Design review of the part built by this model. Coordinates are the model's own, in mm. A direction names the side the tool comes from. Coordinates: 2 decimals unless noted, no trailing zeros. Order: outer loops, then holes, each group sorted by start corner. A loop starts at its lowest first (then second) coordinate and runs counter-clockwise, first axis right, second up. Notation, with made-up numbers: (-6.5, 83) -> (-2.5, 83) arc R20 ccw to (-2.5, 96) -> close; hole circle Ø6 at (27, -20). An arc over 180 degrees is marked (long way). Write item = value, one per line.
```python
from build123d import *

# Parameters (mm, degrees)
F0_W      = 44
F0_H      = 27
F1_DEPTH  = 9
F2_W      = 34
F2_H      = 23
F3_DEPTH  = 7
F6_W      = 6
F6_H      = 7.5
F7_DEPTH  = 4
F5_W      = 6
F5_H      = 7.5
F10_DEPTH = 4
F12_DEPTH = 5
F14_R     = 2
F15_R     = 5


with BuildPart() as f1:
    # F0 (on Top) → F1 (new body)
    with BuildSketch(Plane.XY):
        with Locations((-1, 0)):
            Rectangle(F0_W, F0_H)
    extrude(amount=-F1_DEPTH)


with BuildPart() as f3:
    # F2 (on Top) → F3 (new body)
    with BuildSketch(Plane.XY):
        with Locations((4, 0)):
            Rectangle(F2_W, F2_H)
    extrude(amount=-F3_DEPTH)


with BuildPart() as f1_1:
    add(f1.part)

    # F4: cut F3
    add(f3.part, mode=Mode.SUBTRACT)


with BuildPart() as f7:
    # F6 (on Top) → F7 (new body)
    with BuildSketch(Plane.XY):
        with Locations((-16, -7.75)):
            Rectangle(F6_W, F6_H)
    extrude(amount=-F7_DEPTH)


with BuildPart() as f7b:
    # F5 (on Top) → F7, piece 2 (new body)
    with BuildSketch(Plane.XY):
        with Locations((-16, 7.75)):
            Rectangle(F5_W, F5_H)
    extrude(amount=-F7_DEPTH)


with BuildPart() as f1_2:
    add(f1_1.part)

    # F8: cut F7b, F7
    add(f7b.part, mode=Mode.SUBTRACT)
    add(f7.part, mode=Mode.SUBTRACT)

    # F9 (on face) → F10 (join)
    with BuildSketch(Plane(origin=(-23, 0, 0), x_dir=(0, -1, 0), z_dir=(-1, 0, 0))):
        Polygon((-13.5, 0), (13.5, 0), (33.5, 34.6410161514), (-33.5, 34.6410161514), align=None)
    extrude(amount=-F10_DEPTH)


with BuildPart() as f12:
    # F11 (on face) → F12 (new body)
    with BuildSketch(Plane(origin=(-23, 0, 0), x_dir=(0, -1, 0), z_dir=(-1, 0, 0))):
        Polygon((-7.5, 0), (7.5, 0), (27.5, 34.6410161514), (-27.5, 34.6410161514), align=None)
    extrude(amount=-F12_DEPTH)


with BuildPart() as f1_3:
    add(f1_2.part)

    # F13: cut F12
    add(f12.part, mode=Mode.SUBTRACT)

    # F14
    f14_edges = [f1_3.edges().sort_by_distance(p)[0] for p in [
        (-21, 33.5, 34.641016),
        (-21, 27.5, 34.641016),
        (-21, -27.5, 34.641016),
        (-21, -33.5, 34.641016),
        (-21, -7.5, 0),
        (-21, 7.5, 0),
        (-13, 0, 0),
        (-13, 7.75, -4),
        (-13, -7.75, -4),
    ]]
    fillet(f14_edges, radius=F14_R)

    # F15
    f15_edges = [f1_3.edges().sort_by_distance(p)[0] for p in [
        (-19, -12.5, 0),
        (-19, 12.5, 0),
        (21, 12.5, 0),
        (21, -12.5, 0),
    ]]
    fillet(f15_edges, radius=F15_R)


solid = f1_3.part
```
(1) Insertion check: pin 1 (1.6 mm diameter, centred on x = -4, y = -13, fed in from +Z); pin 2 (3 mm diameter, centred on x = -16.5, y = -9.5, fed in from +Z); pin 3 (1 mm diameter, centred on y = 1, z = -2.5, fed in from +X). Each pin has a flat end and moves straight along its axis. Give the tip position at first contact, or say it passes through.
Report:
pin_1 = 0
pin_2 = -4
pin_3 = -13
(2) For L1, parallel to Y at x = 11, z = -4.5; L2, parallel to Z at x = 6, y = -5; L3, parallel to X at y = -24, z = 26.5, list the stretches that pass through material, from the lowest coordinate up.
Report:
L1 = -13.5 to -11.5, 11.5 to 13.5
L2 = -9 to -7
L3 = -23 to -19
(3) We need section A-A (z = 25.5). Write out the cut boundary in (x, y), and give its area (3 significant figures).
Report:
outline = (-23, -28.22) -> (-19, -28.22) -> (-19, -22.22) -> (-23, -22.22) -> close; (-23, 22.22) -> (-19, 22.22) -> (-19, 28.22) -> (-23, 28.22) -> close
area = 48.0 mm²
(4) We need section B-B (x = -2). Write out the cut boundary in (y, z), and give its area (3 significant figures).
Report:
outline = (-13.5, -9) -> (13.5, -9) -> (13.5, 0) -> (11.5, 0) -> (11.5, -7) -> (-11.5, -7) -> (-11.5, 0) -> (-13.5, 0) -> close
area = 82.0 mm²
(5) We need section D-D (y = -14.5). Write out the cut boundary in (x, z), and give its area (3 significant figures).
Report:
outline = (-23, 1.73) -> (-17.78, 1.73) arc R5 cw to (-19, 5) -> (-19, 12.12) -> (-23, 12.12) -> close
area = 42.8 mm²
(6) We need section C-C (y = 0). Write out the cut boundary in (x, z).
Report:
outline = (-23, -9) -> (21, -9) -> (21, -7) -> (-13, -7) -> (-13, -2) arc R2 ccw to (-15, 0) -> (-23, 0) -> close
(7) The part is to be moulded in two halves that separate along Y. For faces 4 (the cylindrical face through (20, -12, -2)), 5 (the flat face through (-1, -13.5, -4)), 6 (the cylindrical face through (-20.972, -27.642, 34.366)), say which applies: released by +Y, released by -Y, zero draft, split by the parting line, or undercut.
Report:
face_4 = zero draft
face_5 = released by -Y
face_6 = undercut
(8) For faces 1 (the flat face through (-17, 8, -4)), 2 (the flat face through (-21.028, 17.632, 17.549)), 3 (the cylindrical face through (-18, -13, 2)), list the 3-axis set-ups (+Z, -Z, +X, -X, +Y, -Y) from which the entire face can be reached by the end or side of a thin tool; tool diameter is ignored.
Report:
face_1 = +Z, +X
face_2 = +Z, +X, -X
face_3 = +Z, +X, +Y, -Y
